Design review of the part built by this model. Coordinates are the model's own, in mm. Coordinates: 2 decimals unless noted, no trailing zeros. Loops run counter-clockwise (first coordinate to the right, second up) from the corner with the lowest first, then second, coordinate; pieces in that order, holes last.
from build123d import *

# Parameters (mm, degrees)
SKETCH2_W           = 22.42
SKETCH2_H           = 92
BOSS_EXTRUDE2_DEPTH = 0.2
FILLET4_R           = 3
FILLET7_R           = 3
SKETCH4_W           = 2
SKETCH4_H           = 54.51
CUT_EXTRUDE1_DEPTH  = 0.2
SKETCH5_W           = 2
SKETCH5_H           = 54.51
CUT_EXTRUDE2_DEPTH  = 0.2
CUT_EXTRUDE3_DEPTH  = 0.2
CUT_EXTRUDE4_DEPTH  = 0.2
CUT_EXTRUDE7_DEPTH  = 0.2
CUT_EXTRUDE8_DEPTH  = 0.2


with BuildPart() as part:
    # Sketch2 → Boss-Extrude2 (new body)
    with BuildSketch(Plane(origin=(0, 0, 0), x_dir=(0, 1, 0), z_dir=(-1, 0, 0))):
        with Locations((-43.813076923, -17.338461538)):
            Rectangle(SKETCH2_W, SKETCH2_H)
    extrude(amount=BOSS_EXTRUDE2_DEPTH)

    # Fillet4
    fillet4_edges = [part.edges().sort_by_distance(p)[0] for p in [
        (-0.1, -55.023076923, -28.661538462),
    ]]
    fillet(fillet4_edges, radius=FILLET4_R)

    # Fillet7
    fillet7_edges = [part.edges().sort_by_distance(p)[0] for p in [
        (-0.1, -32.603076923, -28.661538462),
    ]]
    fillet(fillet7_edges, radius=FILLET7_R)

    # Sketch4 → Cut-Extrude1 (cut)
    with BuildSketch(Plane(origin=(-0.2, 0, 0), x_dir=(0, 1, 0), z_dir=(-1, 0, 0))):
        with Locations((-54.023076923, -36.083461538)):
            Rectangle(SKETCH4_W, SKETCH4_H)
    extrude(amount=-CUT_EXTRUDE1_DEPTH, mode=Mode.SUBTRACT)

    # Sketch5 → Cut-Extrude2 (cut)
    with BuildSketch(Plane(origin=(-0.2, 0, 0), x_dir=(0, 1, 0), z_dir=(-1, 0, 0))):
        with Locations((-33.603076923, -36.083461538)):
            Rectangle(SKETCH5_W, SKETCH5_H)
    extrude(amount=-CUT_EXTRUDE2_DEPTH, mode=Mode.SUBTRACT)

    # Sketch6 → Cut-Extrude3 (cut)
    with BuildSketch(Plane(origin=(-0.2, 0, 0), x_dir=(0, 1, 0), z_dir=(-1, 0, 0))):
        Polygon((-53.023076923, -63.338461538), (-53.023076923, -61.338461538), (-51.023076923, -63.338461538), align=None)
    extrude(amount=-CUT_EXTRUDE3_DEPTH, mode=Mode.SUBTRACT)

    # Sketch7 → Cut-Extrude4 (cut)
    with BuildSketch(Plane(origin=(-0.2, 0, 0), x_dir=(0, 1, 0), z_dir=(-1, 0, 0))):
        Polygon((-34.603076923, -63.338461538), (-34.603076923, -61.338461538), (-36.603076923, -63.338461538), align=None)
    extrude(amount=-CUT_EXTRUDE4_DEPTH, mode=Mode.SUBTRACT)

    # Sketch8 → Cut-Extrude7 (cut)
    with BuildSketch(Plane(origin=(-0.2, 0, 0), x_dir=(0, 1, 0), z_dir=(-1, 0, 0))):
        Polygon((-53.023076923, -8.828461538), (-55.023076923, -8.828461538), (-55.023076923, -6.828461538), align=None)
    extrude(amount=-CUT_EXTRUDE7_DEPTH, mode=Mode.SUBTRACT)

    # Sketch9 → Cut-Extrude8 (cut)
    with BuildSketch(Plane(origin=(-0.2, 0, 0), x_dir=(0, 1, 0), z_dir=(-1, 0, 0))):
        Polygon((-34.603076923, -8.828461538), (-32.603076923, -8.828461538), (-32.603076923, -6.828461538), align=None)
    extrude(amount=-CUT_EXTRUDE8_DEPTH, mode=Mode.SUBTRACT)


solid = part.part
Q1. Clearance check with a flat-ended pin moving along its axis: pin 1 Ø3 at (y, z) = (-49.5, 46) entering from +X. State where the tip first meets the part, or that it passes through.
Q2. Take a section at A-A, the plane x = -0.1. Write out the cut boundary in (y, z).
Q3. For line 1 (Y direction, x = -0.1, z = 33); line 2 (Z direction, x = -0.1, y = -34.5), list the stretches that pass through material, from the lowest coordinate up.
Q4. Take a section at B-B, the plane z = 23.5. Write out the cut boundary in (x, y).
Entries:
1. pin 1: stops at x = 0
2. outline: (-55.02, -25.66) arc R3 ccw to (-52.02, -28.66) - (-35.6, -28.66) arc R3 ccw to (-32.6, -25.66) - (-32.6, 6.83) - (-34.6, 8.83) - (-34.6, 61.34) - (-36.6, 63.34) - (-51.02, 63.34) - (-53.02, 61.34) - (-53.02, 8.83) - (-55.02, 6.83) - close
3. line 1: y = -53.02 to -34.6
3. line 2: z = -28.45 to 8.73
4. outline: (-0.2, -53.02) - (0, -53.02) - (0, -34.6) - (-0.2, -34.6) - close
